Verification items for this drawing (mm, ordinates from the low corner). A direction names the side the tool comes from. Give positions to 0.01 mm unless a question says otherwise; leave off trailing zeros. Answer as a JSON object with one key per item and string values.
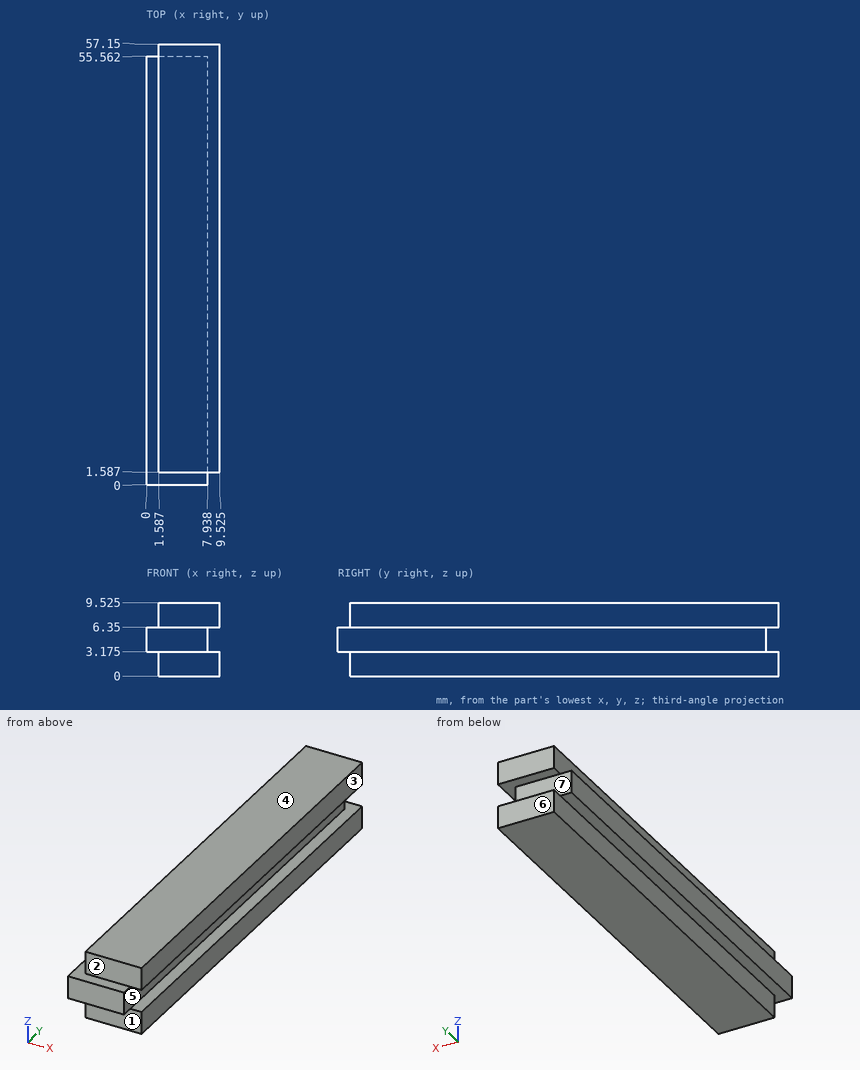
1. Go/stop test with flat-tipped pins: P1, Ø4, axis at x = 1.5, z = 1, coming from the -Y side; P2, Ø2.5, axis at y = 24.5, z = 1, coming from the -X side; P3, Ø1.6, axis at x = 5.5, z = 5.5, coming from the +Y side. Record where each tip stops, or that it passes through.
Determined:
{"P1": "y = 1.59", "P2": "x = 1.59", "P3": "y = 55.56"}
2. Scan lines: L1, parallel to Y at x = 2.75, z = 7.75; L2, parallel to X at y = 28, z = 1 (1 decimal); L3, parallel to X at y = 48, z = 4.5. Record each from-to range of solid material in increasing order. Write a range as [from, to].
Determined:
{"L1": "[1.59, 57.15]", "L2": "[1.6, 9.5]", "L3": "[0, 7.94]"}
3. Mould release check, pull along Z, two halves, no side actions. Record for the marked faces 4, 5, 6 and 7: released by +Z, released by -Z, zero draft, split by the parting line, or undercut.
Determined:
{"face 4": "released by +Z", "face 5": "undercut", "face 6": "zero draft", "face 7": "undercut"}
4. Access from +Z, -Z, +X, -X, +Y, -Y to the whole of each face (thin tool, end or side, straight path). Record for the marked faces 1, 2 and 3.
Determined:
{"face 1": "-Z, +X, -X, -Y", "face 2": "+Z, +X, -X, -Y", "face 3": "+Z, -Z, +X, +Y, -Y"}
